The figure shows three views and two pictorial views of one solid part (mm, origin at its lowest corner). Answer the questions. A direction names the side the tool comes from. Coordinates: 2 decimals unless noted, no trailing zeros. Order: outer loops, then holes, each group sorted by start corner. A loop starts at its lowest first (then second) coordinate and runs counter-clockwise, first axis right, second up. Notation, with made-up numbers: (9.25, 48) - (50.25, 48) arc R20 ccw to (50.25, 85) - close; hole circle Ø4 at (12.5, 72.5). An arc over 180 degrees is marked (long way). Use one line per item in the form item = value. Start each with the question number.
Item 1: Section B-B, the plane x = 9 is taken. Write down the section's boundary in (y, z).
Item 2: Each of these flat-tipped pins is pushed along its axis until it touches: pin 1 Ø2 at (x, y) = (11.5, 2.5) entering from -Z; pin 2 Ø1.9 at (x, y) = (8.5, 4) entering from +Z; pin 3 Ø3 at (y, z) = (2, 18.5) entering from +X; pin 4 Ø5 at (x, y) = (6.5, 3) entering from +Z. Where does it stop, or does it pass through?
Item 3: Section A-A, the plane y = 4 is taken. Write down the section's boundary in (x, z), and give its area (3 significant figures).
Item 4: Consider line 1 along Z through (x, y) = (12, 3); line 2 along Y through (x, z) = (2.15, 14); line 3 along X through (y, z) = (5.25, 4.25). Determine where each line is inside the solid, lowest interval first. Write a range as [from, to].
Item 5: A tool of negligible diameter and unlimited length cuts with its end or side. For the marked faces 1, 2, 3, 4 and 5, from which of +Z, -Z, +X, -X, +Y, -Y can it reach the whole face along a straight path? Write none if from no direction.
Item 6: Section D-D, the plane y = 8.5 is taken. Write down the section's boundary in (x, z).
Item 7: Section C-C, the plane z = 2 is taken. Write down the section's boundary in (x, y), and give its area (3 significant figures).
Item 8: The mould has two halves that part along Z. Classify the marked faces 6, 7 and 8: released by +Z, released by -Z, zero draft, split by the parting line, or undercut.
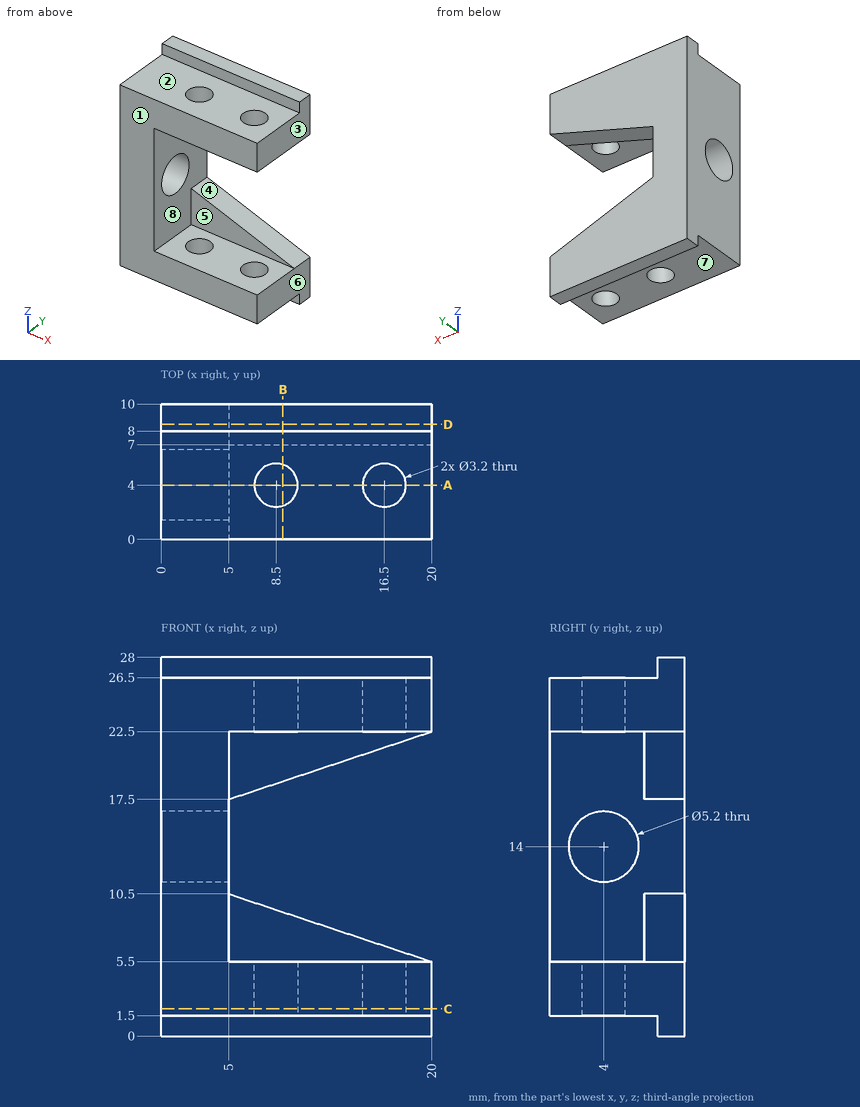
Response:
q1.outline = (0, 1.5) - (2.48, 1.5) - (2.48, 5.5) - (0, 5.5) - close; (0, 22.5) - (2.48, 22.5) - (2.48, 26.5) - (0, 26.5) - close; (5.52, 1.5) - (8, 1.5) - (8, 0) - (10, 0) - (10, 9.17) - (7, 9.17) - (7, 5.5) - (5.52, 5.5) - close; (5.52, 22.5) - (7, 22.5) - (7, 18.83) - (10, 18.83) - (10, 28) - (8, 28) - (8, 26.5) - (5.52, 26.5) - close
q2.pin_1 = 1.5
q2.pin_2 = through
q2.pin_3 = 5
q2.pin_4 = 26.5
q3.outline = (0, 1.5) - (6.9, 1.5) - (6.9, 5.5) - (5, 5.5) - (5, 11.4) - (0, 11.4) - close; (0, 16.6) - (5, 16.6) - (5, 22.5) - (6.9, 22.5) - (6.9, 26.5) - (0, 26.5) - close; (10.1, 1.5) - (14.9, 1.5) - (14.9, 5.5) - (10.1, 5.5) - close; (10.1, 22.5) - (14.9, 22.5) - (14.9, 26.5) - (10.1, 26.5) - close; (18.1, 1.5) - (20, 1.5) - (20, 5.5) - (18.1, 5.5) - close; (18.1, 22.5) - (20, 22.5) - (20, 26.5) - (18.1, 26.5) - close
q3.area = 168 mm2
q4.line_1 = [1.5, 5.5], [22.5, 26.5]
q4.line_2 = [0, 1.4], [6.6, 10]
q4.line_3 = [0, 7.5], [9.5, 15.5], [17.5, 20]
q5.face_1 = +Z, -Z, +X, -X, -Y
q5.face_2 = +Z, +X, -X, -Y
q5.face_3 = +Z, -Z, +X, +Y, -Y
q5.face_4 = +X, +Y, -Y
q5.face_5 = +X, -Y
q6.outline = (0, 0) - (20, 0) - (20, 5.5) - (5, 10.5) - (5, 17.5) - (20, 22.5) - (20, 28) - (0, 28) - close
q7.outline = (0, 0) - (20, 0) - (20, 10) - (0, 10) - close; hole circle Ø3.2 at (8.5, 4); hole circle Ø3.2 at (16.5, 4)
q7.area = 184 mm2
q8.face_6 = zero draft
q8.face_7 = released by -Z
q8.face_8 = undercut
